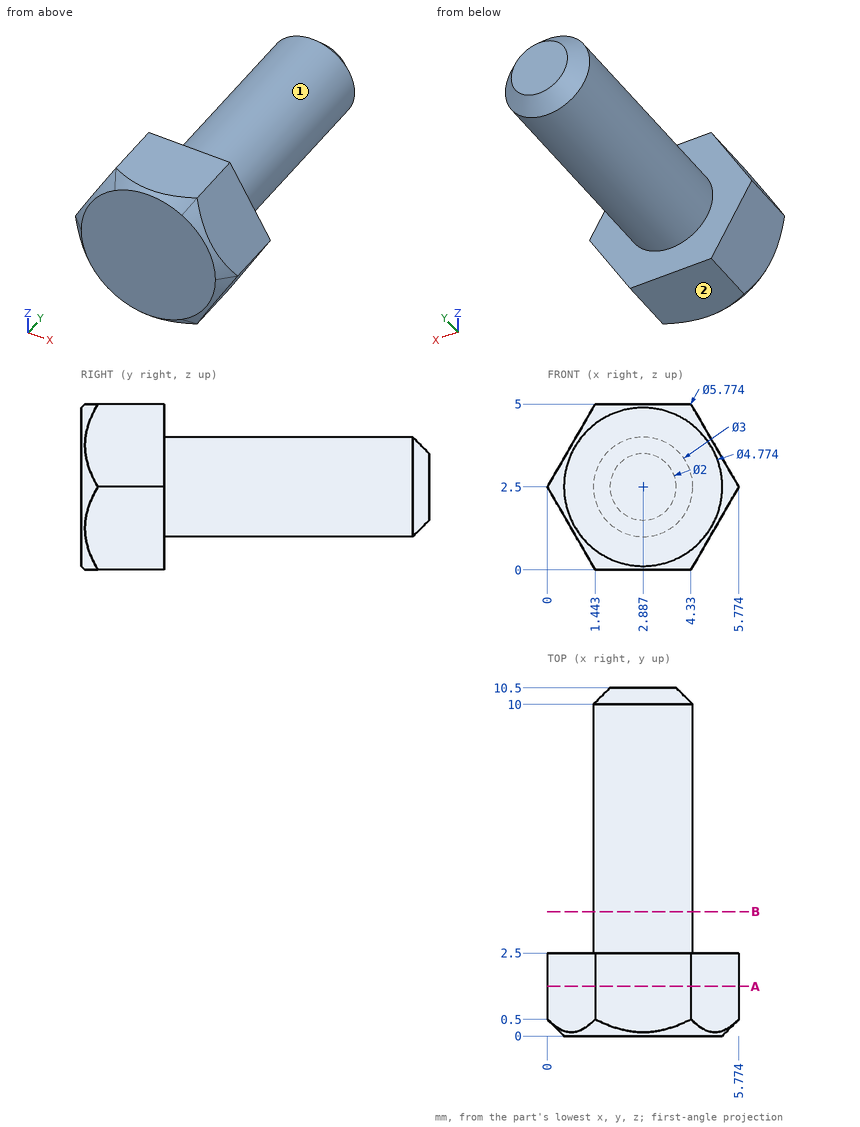
Job drawing, mm, ordinate dimensions from the low corner. One solid piece. A direction names the side the tool comes from. Round coordinates to 2 decimals unless told otherwise and drop trailing zeros. Loops run counter-clockwise (first coordinate to the right, second up) from the corner with the lowest first, then second, coordinate; pieces in that order, holes last. Notation, with made-up numbers: (-26.5, 69) -> (-16.5, 69) arc R14 ccw to (-16.5, 92) -> close; hole circle Ø10 at (79, -27.75). An arc over 180 degrees is marked (long way). Use CSV: the item, a comma, the result in double quotes. Start each with the question number.
Q1. Saw through at B-B on y = 3.75. Give the cut face in (x, z).
Q2. Drill centre lines: L1, parallel to Y at x = 4.65, z = 3.85; L2, parallel to X at y = 6, z = 1.7 (1 decimal); L3, parallel to X at y = 0.5, z = 4.5 (1 decimal). Where is each one in solid material? Low to high.
Q3. Which spindle directions (+Z, -Z, +X, -X, +Y, -Y) get a long thin tool onto all of the face, cutting with end or side? Do the marked faces 1 and 2. Say none if no direction does.
Q4. Flat gauge pin, fed straight in: pin 1 Ø1 at (y, z) = (4, 2) entering from -X. Where does the tip first touch, or does it go through?
Q5. Saw through at A-A on y = 1.5. Give the cut face in (x, z).
Solutions:
1,outline,"circle Ø3 at (2.89, 2.5)"
2,L1,"y = 0 to 2.5"
2,L2,"x = 1.6 to 4.2"
2,L3,"x = 1.2 to 4.6"
3,face 1,"+Y"
3,face 2,"-Z, +X, -X, +Y, -Y"
4,pin 1,"stops at x = 1.39"
5,outline,"(0, 2.5) -> (1.44, 0) -> (4.33, 0) -> (5.77, 2.5) -> (4.33, 5) -> (1.44, 5) -> close"
